```python
from build123d import *

# Parameters (mm, degrees)
EXTRUDE_1_DEPTH     = 150
SKETCH_2_R          = 1.6
CUT_EXTRUDE_1_DEPTH = 151.741633267


with BuildPart() as part:
    # 草图1 → 凸台-拉伸1 (new body)
    with BuildSketch(Plane(origin=(0, 0, 0), x_dir=(1, 0, 0), z_dir=(0, 1, 0))):
        Polygon((0, 0), (0, 1.4), (1, 1.4), (1, 2.9), (0, 2.9), (0, 5.2), (14, 5.2), (14, 2.9), (13, 2.9), (13, 1.4), (14, 1.4), (14, 0), align=None)
    extrude(amount=EXTRUDE_1_DEPTH)

    # 草图2 → 切除-拉伸1 (cut, through all)
    with BuildSketch(Plane(origin=(0, 0, -5.2), x_dir=(-1, 0, 0), z_dir=(0, 0, -1))):
        with Locations((-7, 15)):
            Circle(SKETCH_2_R)
        with Locations((-7, 45)):
            Circle(SKETCH_2_R)
        with Locations((-7, 75)):
            Circle(SKETCH_2_R)
        with Locations((-7, 105)):
            Circle(SKETCH_2_R)
        with Locations((-7, 135)):
            Circle(SKETCH_2_R)
    extrude(amount=-CUT_EXTRUDE_1_DEPTH, mode=Mode.SUBTRACT)


solid = part.part
```
The listing builds one solid part. Answer for the finished solid, in the listing's coordinates (mm). Coordinates: 2 decimals unless noted, no trailing zeros. Order: outer loops, then holes, each group sorted by start corner. A loop starts at its lowest first (then second) coordinate and runs counter-clockwise, first axis right, second up. Notation, with made-up numbers: M 49.25,62 L 91.25,62 A16 cw 91.25,72 Z; hole C 28,30.5 d7. An arc over 180 degrees is marked long. Answer as a JSON object with one key per item and string values. Group by question number.
1. Determine the mould class of faces 1 (the cylindrical face through (7.208, 16.586, -2.636)), 2 (the flat face through (7, 150, -3)), 3 (the flat face through (0, 74, -4)) for opening direction Y: released by +Y, released by -Y, zero draft, split by the parting line, or undercut.
2. Section A-A on y = 75 is taken. Write down the section's boundary in (x, z).
3. Straight lines are drawn through the part: line 1 (Y direction, x = 7, z = -2.6); line 2 (Y direction, x = 6, z = -3.5); line 3 (X direction, y = 75, z = -2.2). For each, find the intervals that lie inside material, in ascending order.
4. Section C-C on y = 51.5 is taken. Write down the section's boundary in (x, z).
5. Section B-B on x = 7 is taken. Write down the section's boundary in (y, z).
6. A flat-ended cylindrical pin translates along its axis: P1, Ø0.8, axis at y = 106, z = -2, coming from the +X side. Find the tip coordinate at first contact, or state that the pin passes through.
Values follow:
{
 "1": {"face 1": "undercut", "face 2": "released by +Y", "face 3": "zero draft"},
 "2": {"outline": "M 0,-5.2 L 5.4,-5.2 L 5.4,0 L 0,0 L 0,-1.4 L 1,-1.4 L 1,-2.9 L 0,-2.9 Z; M 8.6,-5.2 L 14,-5.2 L 14,-2.9 L 13,-2.9 L 13,-1.4 L 14,-1.4 L 14,0 L 8.6,0 Z"},
 "3": {"line 1": "0 to 13.4, 16.6 to 43.4, 46.6 to 73.4, 76.6 to 103.4, 106.6 to 133.4, 136.6 to 150", "line 2": "0 to 13.75, 16.25 to 43.75, 46.25 to 73.75, 76.25 to 103.75, 106.25 to 133.75, 136.25 to 150", "line 3": "1 to 5.4, 8.6 to 13"},
 "4": {"outline": "M 0,-5.2 L 14,-5.2 L 14,-2.9 L 13,-2.9 L 13,-1.4 L 14,-1.4 L 14,0 L 0,0 L 0,-1.4 L 1,-1.4 L 1,-2.9 L 0,-2.9 Z"},
 "5": {"outline": "M 0,-5.2 L 13.4,-5.2 L 13.4,0 L 0,0 Z; M 16.6,-5.2 L 43.4,-5.2 L 43.4,0 L 16.6,0 Z; M 46.6,-5.2 L 73.4,-5.2 L 73.4,0 L 46.6,0 Z; M 76.6,-5.2 L 103.4,-5.2 L 103.4,0 L 76.6,0 Z; M 106.6,-5.2 L 133.4,-5.2 L 133.4,0 L 106.6,0 Z; M 136.6,-5.2 L 150,-5.2 L 150,0 L 136.6,0 Z"},
 "6": {"P1": "x = 13"}
}
